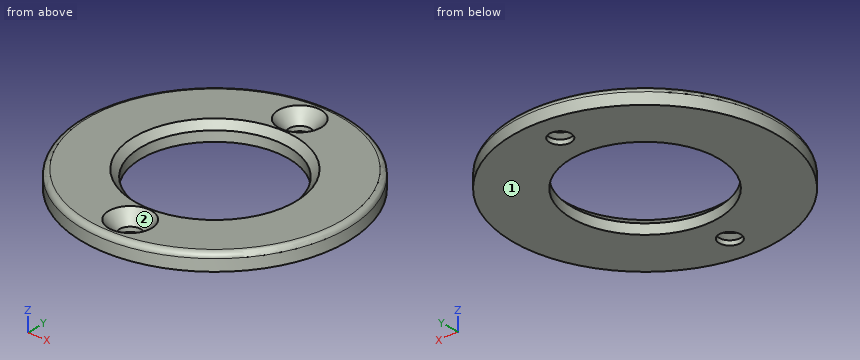
from build123d import *

# Parameters (mm, degrees)
SKETCH1_R                                     = 19.939
BOSS_EXTRUDE1_DEPTH                           = 2.54
F_7_8_0_875_DIAMETER_HOLE1_D                  = 22.225
CSK_FOR_4_FLAT_HEAD_SOCKET_CAP_SCREW1_A_COUNT = 2
CSK_FOR_4_FLAT_HEAD_SOCKET_CAP_SCREW1_A_PITCH = 31.0515
CHAMFER1_SIZE                                 = 1.016
FILLET1_R                                     = 0.79375


with BuildPart() as part:
    # Sketch1 → Boss-Extrude1 (new body)
    with BuildSketch(Plane.XY):
        Circle(SKETCH1_R)
    extrude(amount=BOSS_EXTRUDE1_DEPTH)

    # 7/8 (0.875) Diameter Hole1 (through all)
    with Locations(Plane.XY.offset(2.54)):
        with Locations((0, 0)):
            Hole(F_7_8_0_875_DIAMETER_HOLE1_D / 2)

    # Sketch24 → CSK for #4 Flat Head Socket Cap Screw1 (revolve, cut)
    with BuildSketch(Plane(origin=(0, 15.52575, 2.54), x_dir=(0, -1, 0), z_dir=(1, 0, 0))):
        Polygon((0, 0), (0, 2.54), (1.63195, 2.54), (1.63195, 1.848124365), (3.2385, 0), align=None)
    csk_for_4_flat_head_socket_cap_screw1 = revolve(axis=Axis((0, 15.52575, 8.89), (0, 0, -1)), mode=Mode.SUBTRACT)

    # CSK for #4 Flat Head Socket Cap Screw1 a: CSK for #4 Flat Head Socket Cap Screw1 ×2
    with Locations(*[(0, -i * CSK_FOR_4_FLAT_HEAD_SOCKET_CAP_SCREW1_A_PITCH, 0) for i in range(1, CSK_FOR_4_FLAT_HEAD_SOCKET_CAP_SCREW1_A_COUNT)]):
        add(csk_for_4_flat_head_socket_cap_screw1, mode=Mode.SUBTRACT)

    # Chamfer1
    chamfer1_edges = [part.edges().sort_by_distance(p)[0] for p in [
        (11.1125, 0, 2.54),
    ]]
    chamfer(chamfer1_edges, length=CHAMFER1_SIZE)

    # Fillet1
    fillet1_edges = [part.edges().sort_by_distance(p)[0] for p in [
        (-19.939, 0, 2.54),
    ]]
    fillet(fillet1_edges, radius=FILLET1_R)


solid = part.part
Work out the finished part from the listing and answer in its coordinate system (mm). Face numbers are marked on the shaded views. Give positions to 0.01 mm unless a question says otherwise; leave off trailing zeros. Write each loop counter-clockwise with the first axis right and the second up, starting at its lowest first coordinate (ties: lowest second). Pieces come first, ordered by that corner, then holes.
Q1. For a pull along Y with two mould halves and no side action, classify the marked faces 1 and 2 as released by +Y, released by -Y, zero draft, split by the parting line, or undercut.
Answer:
face 1: zero draft
face 2: undercut
Q2. Straight lines are drawn through the part: L1, parallel to Y at x = 0, z = 0.5; L2, parallel to X at y = -5, z = 1.3; L3, parallel to X at y = -15.5, z = 2.25. For each, find the intervals that lie inside material, in ascending order.
Answer:
L1: y = -19.94 to -17.16, -13.89 to -11.11, 11.11 to 13.89, 17.16 to 19.94
L2: x = -19.3 to -9.92, 9.92 to 19.3
L3: x = -12.25 to -2.99, 2.99 to 12.25
Q3. The part is cut by section B-B on y = 0. Give the vertices of the cut face in (x, z), and give its area (3 significant figures).
Answer:
outline: (-19.94, 0) - (-11.11, 0) - (-11.11, 1.52) - (-12.13, 2.54) - (-19.15, 2.54) arc R0.79 ccw to (-19.94, 1.75) - close; (11.11, 0) - (19.94, 0) - (19.94, 1.75) arc R0.79 ccw to (19.15, 2.54) - (12.13, 2.54) - (11.11, 1.52) - close
area: 43.5 mm2
Q4. Given pin 1 (1.5 mm diameter, centred on y = -7.5, z = 0.5, fed in from -X), flat-ended and moving along its own axis, determine where the tip first touches the part or whether it passes through.
Answer:
pin 1: stops at x = -18.76
Q5. The part is cut by section A-A on x = 0. Give the vertices of the cut face in (y, z).
Answer:
outline: (-19.94, 0) - (-17.16, 0) - (-17.16, 0.69) - (-18.76, 2.54) - (-19.15, 2.54) arc R0.79 ccw to (-19.94, 1.75) - close; (-13.89, 0) - (-11.11, 0) - (-11.11, 1.52) - (-12.13, 2.54) - (-12.29, 2.54) - (-13.89, 0.69) - close; (11.11, 0) - (13.89, 0) - (13.89, 0.69) - (12.29, 2.54) - (12.13, 2.54) - (11.11, 1.52) - close; (17.16, 0) - (19.94, 0) - (19.94, 1.75) arc R0.79 ccw to (19.15, 2.54) - (18.76, 2.54) - (17.16, 0.69) - close
